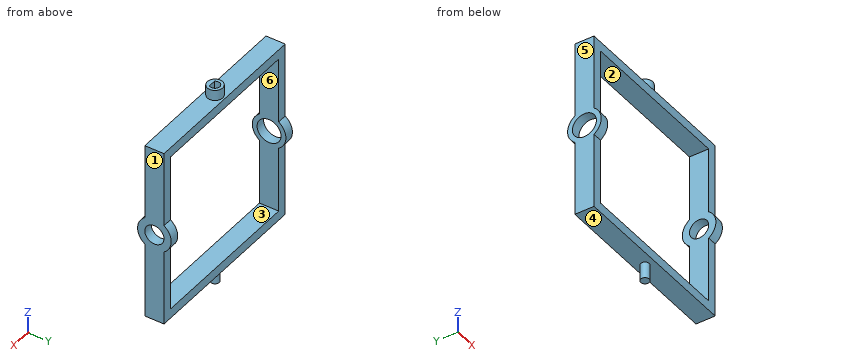
Autodesk Inventor part; units mm, degrees
ref_plane "YZ Plane" through (0, 0, 0) normal (1, 0, 0) x (0, 1, 0)
ref_plane "XZ Plane" through (0, 0, 0) normal (0, 1, 0) x (-1, 0, 0)
ref_plane "XY Plane" through (0, 0, 0) normal (0, 0, 1) x (1, 0, 0)
sketch "Sketch1" plane through (0, 0, 0) normal (0, 1, 0) x (-1, 0, 0)
  line L0 (-52.705, 52.705) -> (52.705, 52.705)
  line L1 (52.705, 52.705) -> (52.705, -52.705)
  line L2 (52.705, -52.705) -> (-52.705, -52.705)
  line L3 (-52.705, -52.705) -> (-52.705, 52.705)
  line L4 (-52.705, 52.705) -> (52.705, -52.705) construction
  line L5 (52.705, 52.705) -> (-52.705, -52.705) construction
  line L6 (-59.055, 59.055) -> (59.055, 59.055)
  line L7 (59.055, 59.055) -> (59.055, -59.055)
  line L8 (59.055, -59.055) -> (-59.055, -59.055)
  line L9 (-59.055, -59.055) -> (-59.055, 59.055)
  line L10 (-59.055, 59.055) -> (59.055, -59.055) construction
  line L11 (59.055, 59.055) -> (-59.055, -59.055) construction
  point P0 (0, 0)
  dimension "d0" = 105.41
  dimension "d1" = 105.41
  dimension "d2" = 118.11
  dimension "d3" = 118.11
extrude "Extrusion1" add sketch "Sketch1" along normal blind 12.7
sketch "Sketch2" plane through (-59.055, 0, -59.055) normal (-1, 0, 0) x (0, 0, 1)
  circle A0 centre (59.055, 6.35) radius 11.1125
  line L0 (0, 0) -> (0, 12.7) construction
  line L1 (0, 6.35) -> (59.055, 6.35) construction
  line L2 (59.055, 6.35) -> (118.11, 6.35) construction
  line L3 (118.11, 0) -> (118.11, 12.7) construction
  point P0 (59.055, 0)
  dimension "d6" = 22.225
extrude "Extrusion2" add sketch "Sketch2" against normal up to surface (6.35 mm away)
sketch "Sketch3" plane through (-59.055, 0, -59.055) normal (-1, 0, 0) x (0, 0, 1)
  circle A0 centre (59.055, 6.35) radius 7.9375
  line L0 (0, 0) -> (0, 12.7) construction
  line L1 (0, 6.35) -> (59.055, 6.35) construction
  line L2 (59.055, 6.35) -> (118.11, 6.35) construction
  line L3 (118.11, 0) -> (118.11, 12.7) construction
  point P0 (59.055, 0)
  dimension "d9" = 15.875
extrude "Extrusion3" cut sketch "Sketch3" against normal up to next
sketch "Sketch4" plane through (59.055, 0, 59.055) normal (1, 0, 0) x (0, 0, -1)
  circle A0 centre (59.055, 6.35) radius 11.1125
  line L0 (0, 0) -> (0, 12.7) construction
  line L1 (0, 6.35) -> (59.055, 6.35) construction
  line L2 (59.055, 6.35) -> (118.11, 6.35) construction
  line L3 (118.11, 0) -> (118.11, 12.7) construction
  point P0 (59.055, 0)
  dimension "d24" = 22.225
extrude "Extrusion4" add sketch "Sketch4" against normal up to surface (6.35 mm away)
sketch "Sketch5" plane through (59.055, 0, 59.055) normal (1, 0, 0) x (0, 0, -1)
  circle A0 centre (59.055, 6.35) radius 6.35
  line L0 (0, 0) -> (0, 12.7) construction
  line L1 (0, 6.35) -> (59.055, 6.35) construction
  line L2 (59.055, 6.35) -> (118.11, 6.35) construction
  line L3 (118.11, 0) -> (118.11, 12.7) construction
  point P0 (59.055, 0)
  dimension "d14" = 12.7
extrude "Extrusion5" cut sketch "Sketch5" against normal up to next
sketch "Sketch6" plane through (59.055, 0, -59.055) normal (0, 0, -1) x (-1, 0, 0)
  circle A0 centre (59.055, 6.35) radius 2.794
  line L0 (0, 0) -> (0, 12.7) construction
  line L1 (0, 6.35) -> (59.055, 6.35) construction
  line L2 (59.055, 6.35) -> (118.11, 6.35) construction
  line L3 (118.11, 14.2875) -> (118.11, -1.5875) construction
  point P0 (59.055, 0)
  dimension "d17" = 5.588
extrude "Extrusion6" add sketch "Sketch6" along normal blind 10.795
sketch "Sketch7" plane through (-59.055, 0, 59.055) normal (0, 0, 1) x (1, 0, 0)
  arc A0 (61.5154, 4.3432) -> (56.5946, 4.3432) centre (59.055, 6.35) ccw
  circle A1 centre (59.055, 6.35) radius 5.08
  line L0 (56.5946, 4.3432) -> (61.5154, 4.3432)
  line L1 (118.11, 0) -> (118.11, 12.7) construction
  line L2 (118.11, 6.35) -> (59.055, 6.35) construction
  line L3 (59.055, 6.35) -> (0, 6.35) construction
  line L4 (0, 0) -> (0, 12.7) construction
  point P0 (59.055, 0)
  dimension "d20" = 6.35
  dimension "d21" = 10.16
extrude "Extrusion7" add sketch "Sketch7" along normal blind 6.985
properties part number "joystick_outer"
Verification items for the finished model (mm, model axes). Face numbers are marked on the shaded views. A direction names the side the tool comes from. Coordinates: 2 decimals unless noted, no trailing zeros. Order: outer loops, then holes, each group sorted by start corner. A loop starts at its lowest first (then second) coordinate and runs counter-clockwise, first axis right, second up. Notation, with made-up numbers: (39.25, 1.25) -> (47.25, 1.25) arc R25 ccw to (47.25, 29.25) -> close; hole circle Ø9 at (-30, 71.25). An arc over 180 degrees is marked (long way). Put each result on its own line as item: value. Start each with the question number.
1. Material ranges on L1, parallel to Z at x = 47.5, y = 1 (3 decimals); L2, parallel to Z at x = 53, y = 2.5 (3 decimals), recorded low to high. Write a range as [from, to].
2. Cross-section at B-B, the plane z = 0. Record the boundary of the cut face in (x, y) (1 decimal), then the cut area to 3 significant figures.
3. Cross-section at D-D, the plane z = 42.5. Record the boundary of the cut face in (x, y) (3 decimals), then the cut area to 3 significant figures.
4. Mould release check, pull along X, two halves, no side actions. Record for the marked faces 3, 4, 5 and 6: released by +X, released by -X, zero draft, split by the parting line, or undercut.
5. Go/stop test with flat-tipped pins: pin 1 Ø15 at (x, z) = (-25, 38) entering from -Y; pin 2 Ø25 at (x, z) = (-8, -45) entering from -Y; pin 3 Ø6 at (x, y) = (16.5, 10.5) entering from -Z (3 decimals); pin 4 Ø1.5 at (x, y) = (-45, 8) entering from +Z (3 decimals). Record where each tip stops, or that it passes through.
6. Access from +Z, -Z, +X, -X, +Y, -Y to the whole of each face (thin tool, end or side, straight path). Record for the marked faces 1 and 2.
7. Cross-section at A-A, the plane x = 0. Record the boundary of the cut face in (y, z) (3 decimals), then the cut area to 3 significant figures.
Computed:
1. L1: [-59.055, -52.705], [52.705, 59.055]
1. L2: [-59.055, -5.05], [5.05, 59.055]
2. outline: (-59.1, -4.8) -> (-52.7, -4.8) -> (-52.7, -1.6) -> (-59.1, -1.6) -> close; (-59.1, 14.3) -> (-52.7, 14.3) -> (-52.7, 17.5) -> (-59.1, 17.5) -> close; (52.7, -4.8) -> (59.1, -4.8) -> (59.1, 0) -> (52.7, 0) -> close; (52.7, 12.7) -> (59.1, 12.7) -> (59.1, 17.5) -> (52.7, 17.5) -> close
2. area: 101 mm2
3. outline: (-59.055, 0) -> (-52.705, 0) -> (-52.705, 12.7) -> (-59.055, 12.7) -> close; (52.705, 0) -> (59.055, 0) -> (59.055, 12.7) -> (52.705, 12.7) -> close
3. area: 161 mm2
4. face 3: undercut
4. face 4: zero draft
4. face 5: released by -X
4. face 6: undercut
5. pin 1: through
5. pin 2: y = 0
5. pin 3: z = -59.055
5. pin 4: z = 59.055
6. face 1: +Z, -Z, +X, +Y, -Y
6. face 2: +Y, -Y
7. outline: (0, -59.055) -> (3.556, -59.055) -> (3.556, -69.85) -> (9.144, -69.85) -> (9.144, -59.055) -> (12.7, -59.055) -> (12.7, -52.705) -> (0, -52.705) -> close; (0, 52.705) -> (12.7, 52.705) -> (12.7, 59.055) -> (11.43, 59.055) -> (11.43, 66.04) -> (9.525, 66.04) -> (9.525, 59.055) -> (4.343, 59.055) -> (4.343, 66.04) -> (1.27, 66.04) -> (1.27, 59.055) -> (0, 59.055) -> close
7. area: 256 mm2
